CAD build for the part. Positions are in the model's coordinates, mm. A direction names the side the tool comes from. Give positions to 0.01 mm unless a question says otherwise; leave off trailing zeros. Order: outer loops, then holes, each group sorted by start corner. A loop starts at its lowest first (then second) coordinate and runs counter-clockwise, first axis right, second up. Notation, with made-up numbers: (6.5, -36.5) -> (48.5, -36.5) arc R34 ccw to (48.5, -3.5) -> close; hole circle Ø9 at (25, 33). An arc over 180 degrees is marked (long way). Answer as CSV lines item,"result".
```python
from build123d import *

# Parameters (mm, degrees)
SKETCH1_R           = 2.5
BOSS_EXTRUDE1_DEPTH = 3
SKETCH1_3_R         = 3
BOSS_EXTRUDE2_DEPTH = 1.5
CHAMFER1_SIZE       = 0.5
CHAMFER3_SIZE       = 0.1


with BuildPart() as part:
    # Sketch1 → Boss-Extrude1 (new, symmetric)
    with BuildSketch(Plane.XY):
        with BuildLine():
            Line((-31, -6), (31, -6))
            ThreePointArc((31, -6), (37, 0), (31, 6))
            Line((31, 6), (-31, 6))
            ThreePointArc((-31, 6), (-37, 0), (-31, -6))
        make_face()
        with Locations((31, 0)):
            Circle(SKETCH1_R, mode=Mode.SUBTRACT)
        with Locations((-31, 0)):
            Circle(SKETCH1_R, mode=Mode.SUBTRACT)
        with BuildLine():
            ThreePointArc((26.641101056, -4.75), (27.549994316, -4.167028828), (27.399170438, -3.097826087))
            ThreePointArc((27.399170438, -3.097826087), (26.25, 0), (27.399170438, 3.097826087))
            ThreePointArc((27.399170438, 3.097826087), (27.549994316, 4.167028828), (26.641101056, 4.75))
            Line((26.641101056, 4.75), (-26.641101056, 4.75))
            ThreePointArc((-26.641101056, 4.75), (-27.549994316, 4.167028828), (-27.399170438, 3.097826087))
            ThreePointArc((-27.399170438, 3.097826087), (-26.25, 0), (-27.399170438, -3.097826087))
            ThreePointArc((-27.399170438, -3.097826087), (-27.549994316, -4.167028828), (-26.641101056, -4.75))
            Line((-26.641101056, -4.75), (26.641101056, -4.75))
        make_face(mode=Mode.SUBTRACT)
    extrude(amount=BOSS_EXTRUDE1_DEPTH, both=True)

    # Sketch1<3> → Boss-Extrude2 (add, symmetric)
    with BuildSketch(Plane.XY):
        with BuildLine():
            Line((-26.641101056, -4.75), (26.641101056, -4.75))
            ThreePointArc((26.641101056, -4.75), (27.549994316, -4.167028828), (27.399170438, -3.097826087))
            ThreePointArc((27.399170438, -3.097826087), (26.25, 0), (27.399170438, 3.097826087))
            ThreePointArc((27.399170438, 3.097826087), (27.549994316, 4.167028828), (26.641101056, 4.75))
            Line((26.641101056, 4.75), (-26.641101056, 4.75))
            ThreePointArc((-26.641101056, 4.75), (-27.549994316, 4.167028828), (-27.399170438, 3.097826087))
            ThreePointArc((-27.399170438, 3.097826087), (-26.25, 0), (-27.399170438, -3.097826087))
            ThreePointArc((-27.399170438, -3.097826087), (-27.549994316, -4.167028828), (-26.641101056, -4.75))
        make_face()
        Circle(SKETCH1_3_R, mode=Mode.SUBTRACT)
        with Locations((10, 0)):
            Circle(SKETCH1_3_R, mode=Mode.SUBTRACT)
        with Locations((20, 0)):
            Circle(SKETCH1_3_R, mode=Mode.SUBTRACT)
        with Locations((-10, 0)):
            Circle(SKETCH1_3_R, mode=Mode.SUBTRACT)
        with Locations((-20, 0)):
            Circle(SKETCH1_3_R, mode=Mode.SUBTRACT)
    extrude(amount=BOSS_EXTRUDE2_DEPTH, both=True)

    # Chamfer1
    chamfer1_edges = [part.edges().sort_by_distance(p)[0] for p in [
        (-37, 0, -3),
        (0, 6, -3),
        (37, 0, -3),
        (0, -6, -3),
        (0, -6, 3),
        (37, 0, 3),
        (0, 6, 3),
        (-37, 0, 3),
    ]]
    chamfer(chamfer1_edges, length=CHAMFER1_SIZE)

    # Chamfer3
    chamfer3_edges = [part.edges().sort_by_distance(p)[0] for p in [
        (-33.5, 0, -3),
        (28.5, 0, -3),
        (28.5, 0, 3),
        (-33.5, 0, 3),
        (-23, 0, 1.5),
        (-13, 0, 1.5),
        (17, 0, 1.5),
        (7, 0, 1.5),
        (-3, 0, 1.5),
        (-3, 0, -1.5),
        (7, 0, -1.5),
        (17, 0, -1.5),
        (-13, 0, -1.5),
        (-23, 0, -1.5),
    ]]
    chamfer(chamfer3_edges, length=CHAMFER3_SIZE)


solid = part.part
```
1) Which spindle directions (+Z, -Z, +X, -X, +Y, -Y) get a long thin tool onto all of the face, cutting with end or side? Do faces 4 (the cylindrical face through (17, 0, 0)), 5 (the cylindrical face through (26.25, -0.05, 2.26)), 6 (the cylindrical face through (-27.557, -4.152, -2.24)). Say none if no direction does.
Data:
face 4,"+Z, -Z"
face 5,"+Z"
face 6,"-Z"
2) Band-saw the part on B-B, the plane z = -0.75. Write the cut outline in (x, y).
Data:
outline,"(-31, -6) -> (31, -6) arc R6 ccw to (31, 6) -> (-31, 6) arc R6 ccw to start; hole circle Ø5 at (-31, 0); hole circle Ø6 at (-20, 0); hole circle Ø6 at (-10, 0); hole circle Ø6 at (0, 0); hole circle Ø6 at (10, 0); hole circle Ø6 at (20, 0); hole circle Ø5 at (31, 0)"
3) Pin check, flat tips, straight feed: P1, Ø2, axis at x = 24.5, y = -1.5, coming from the +Z side; P2, Ø4, axis at x = -31, y = 0, coming from the -Z side; P3, Ø1, axis at x = -14, y = 2, coming from the -Z side; P4, Ø1.5, axis at y = 3, z = 0.5, coming from the +X side. Stop position of each tip, or through.
Data:
P1,"stops at z = 1.5"
P2,"passes through"
P3,"stops at z = -1.5"
P4,"stops at x = 36.56"
4) Wall check: line 1 along Y through (x, z) = (-20, 0.6); line 2 along Y through (x, z) = (-31, -1); line 3 along Z through (x, y) = (-20, 3.5). Give the ranges that are in metal, low to high. Write a range as [from, to].
Data:
line 1,"y = [-6, -3], [3, 6]"
line 2,"y = [-6, -2.5], [2.5, 6]"
line 3,"z = [-1.5, 1.5]"
5) Band-saw the part on A-A, the plane x = 20. Write the cut outline in (y, z).
Data:
outline,"(-6, -2.5) -> (-5.5, -3) -> (-4.75, -3) -> (-4.75, -1.5) -> (-3.1, -1.5) -> (-3, -1.4) -> (-3, 1.4) -> (-3.1, 1.5) -> (-4.75, 1.5) -> (-4.75, 3) -> (-5.5, 3) -> (-6, 2.5) -> close; (3, -1.4) -> (3.1, -1.5) -> (4.75, -1.5) -> (4.75, -3) -> (5.5, -3) -> (6, -2.5) -> (6, 2.5) -> (5.5, 3) -> (4.75, 3) -> (4.75, 1.5) -> (3.1, 1.5) -> (3, 1.4) -> close"
6) Pull direction X, two halves, no side cores. Call faces 1 (the cylindrical face through (-26.25, 0.05, -2.24)), 2 (the conical face through (-36.64, 0.12, -2.86)), 3 (the conical face through (36.634, -0.124, 2.865)): pulls with the +X half, pulls with the -X half, needs draft (parallel to the pull), parting line crosses it, or undercut.
Data:
face 1,"undercut"
face 2,"pulls with the -X half"
face 3,"pulls with the +X half"
7) Band-saw the part on C-C, the plane y = 0. Give the number of separate pieces and of enclosed holes in the cut face, then the cut area to 3 significant figures.
Data:
separate pieces,"8"
enclosed holes,"0"
area,"136 mm2"
